```python
from build123d import *

# Parameters (mm, degrees)
SKETCH1_W           = 15
SKETCH1_H           = 4
BOSS_EXTRUDE1_DEPTH = 1
BOSS_EXTRUDE2_START = 6
BOSS_EXTRUDE2_DEPTH = 6
SKETCH3_W           = 10
SKETCH3_H           = 3
BOSS_EXTRUDE3_DEPTH = 3.5
BOSS_EXTRUDE4_START = 0.6
BOSS_EXTRUDE4_DEPTH = 0.6
SKETCH5_W           = 3
SKETCH5_H           = 10
BOSS_EXTRUDE5_DEPTH = 3.5


with BuildPart() as part:
    # Sketch1 → Boss-Extrude1 (new body)
    with BuildSketch(Plane(origin=(0, 0, 0), x_dir=(1, 0, 0), z_dir=(0, 1, 0))):
        with BuildLine():
            Line((-28, -26.5), (28, -26.5))
            ThreePointArc((28, -26.5), (35.071067812, -23.571067812), (38, -16.5))
            Line((38, -16.5), (38, 16.5))
            ThreePointArc((38, 16.5), (35.071067812, 23.571067812), (28, 26.5))
            Line((28, 26.5), (-28, 26.5))
            ThreePointArc((-28, 26.5), (-35.071067812, 23.571067812), (-38, 16.5))
            Line((-38, 16.5), (-38, -16.5))
            ThreePointArc((-38, -16.5), (-35.071067812, -23.571067812), (-28, -26.5))
        make_face()
        with Locations((16.5, 7)):
            Rectangle(SKETCH1_W, SKETCH1_H, mode=Mode.SUBTRACT)
    extrude(amount=BOSS_EXTRUDE1_DEPTH)

    # Sketch2 → Boss-Extrude2 (add)
    with BuildSketch(Plane.XZ.offset(BOSS_EXTRUDE2_START)):
        with BuildLine():
            Line((-28, -26.5), (28, -26.5))
            ThreePointArc((28, -26.5), (35.071067812, -23.571067812), (38, -16.5))
            Line((38, -16.5), (38, 16.5))
            ThreePointArc((38, 16.5), (35.071067812, 23.571067812), (28, 26.5))
            Line((28, 26.5), (-28, 26.5))
            ThreePointArc((-28, 26.5), (-35.071067812, 23.571067812), (-38, 16.5))
            Line((-38, 16.5), (-38, -16.5))
            ThreePointArc((-38, -16.5), (-35.071067812, -23.571067812), (-28, -26.5))
        make_face()
        with BuildLine():
            Line((28, 25.5), (-28, 25.5))
            ThreePointArc((-28, 25.5), (-34.363961031, 22.863961031), (-37, 16.5))
            Line((-37, 16.5), (-37, -16.5))
            ThreePointArc((-37, -16.5), (-34.363961031, -22.863961031), (-28, -25.5))
            Line((-28, -25.5), (28, -25.5))
            ThreePointArc((28, -25.5), (34.363961031, -22.863961031), (37, -16.5))
            Line((37, -16.5), (37, 16.5))
            ThreePointArc((37, 16.5), (34.363961031, 22.863961031), (28, 25.5))
        make_face(mode=Mode.SUBTRACT)
    extrude(amount=-BOSS_EXTRUDE2_DEPTH)

    # Sketch3 → Boss-Extrude3 (add)
    with BuildSketch(Plane.XZ):
        with Locations((0, -24)):
            Rectangle(SKETCH3_W, SKETCH3_H)
        with Locations((0, 24)):
            Rectangle(SKETCH3_W, SKETCH3_H)
    extrude(amount=BOSS_EXTRUDE3_DEPTH)

    # Sketch4 → Boss-Extrude4 (add)
    with BuildSketch(Plane.XZ.offset(6).offset(BOSS_EXTRUDE4_START)):
        with BuildLine():
            Line((-28, -26.5), (28, -26.5))
            ThreePointArc((28, -26.5), (35.071067812, -23.571067812), (38, -16.5))
            Line((38, -16.5), (38, 16.5))
            ThreePointArc((38, 16.5), (35.071067812, 23.571067812), (28, 26.5))
            Line((28, 26.5), (-28, 26.5))
            ThreePointArc((-28, 26.5), (-35.071067812, 23.571067812), (-38, 16.5))
            Line((-38, 16.5), (-38, -16.5))
            ThreePointArc((-38, -16.5), (-35.071067812, -23.571067812), (-28, -26.5))
        make_face()
        with BuildLine():
            Line((28, 25), (-28, 25))
            ThreePointArc((-28, 25), (-34.01040764, 22.51040764), (-36.5, 16.5))
            Line((-36.5, 16.5), (-36.5, -16.5))
            ThreePointArc((-36.5, -16.5), (-34.01040764, -22.51040764), (-28, -25))
            Line((-28, -25), (28, -25))
            ThreePointArc((28, -25), (34.01040764, -22.51040764), (36.5, -16.5))
            Line((36.5, -16.5), (36.5, 16.5))
            ThreePointArc((36.5, 16.5), (34.01040764, 22.51040764), (28, 25))
        make_face(mode=Mode.SUBTRACT)
    extrude(amount=-BOSS_EXTRUDE4_DEPTH)

    # Sketch5 → Boss-Extrude5 (add)
    with BuildSketch(Plane.XZ):
        with Locations((35.5, 0)):
            Rectangle(SKETCH5_W, SKETCH5_H)
        with Locations((-35.5, 0)):
            Rectangle(SKETCH5_W, SKETCH5_H)
    extrude(amount=BOSS_EXTRUDE5_DEPTH)


solid = part.part
```
Part model, mm, in its own coordinate system. A direction names the side the tool comes from. Round coordinates to 2 decimals unless told otherwise and drop trailing zeros. Write each loop counter-clockwise with the first axis right and the second up, starting at its lowest first coordinate (ties: lowest second). Pieces come first, ordered by that corner, then holes.
Item 1: Probe L1, parallel to Z at x = -23.5, y = -3.75; L2, parallel to X at y = -3.5, z = -8; L3, parallel to X at y = -3, z = -3.5. List the from-to ranges inside material, lowest first.
Results:
L1: z = -26.5 to -25.5, 25.5 to 26.5
L2: x = -38 to -37, 37 to 38
L3: x = -38 to -34, 34 to 38
Item 2: Cut at C-C, the plane x = 17.5. Give the cut face in (y, z).
Results:
outline: (-6.6, -26.5) - (1, -26.5) - (1, -9) - (0, -9) - (0, -25.5) - (-6, -25.5) - (-6, -25) - (-6.6, -25) - close; (-6.6, 25) - (-6, 25) - (-6, 25.5) - (0, 25.5) - (0, -5) - (1, -5) - (1, 26.5) - (-6.6, 26.5) - close
Item 3: Cut at D-D, the plane z = 7. Give the cut face in (x, y).
Results:
outline: (-38, -6.6) - (-36.5, -6.6) - (-36.5, -6) - (-37, -6) - (-37, 0) - (37, 0) - (37, -6) - (36.5, -6) - (36.5, -6.6) - (38, -6.6) - (38, 1) - (-38, 1) - close
Item 4: Two-plate mould, pull along X, no slides. Class faces 4 (the flat face through (-9, -6.6, 26)), 5 (the cylindrical face through (33.94, -6.3, -22.58)), 6 (the cylindrical face through (-34.99, -2.85, 23.65)): +X half, -X half, draft (parallel to the pull), parting line (faces both ways), or undercut.
Results:
face 4: draft
face 5: undercut
face 6: -X half
Item 5: Drop flat-ended pins along their axis: pin 1 Ø2.5 at (x, y) = (-35.5, -2) entering from +Z; pin 2 Ø1.5 at (y, z) = (-1, -23.5) entering from +X; pin 3 Ø0.9 at (y, z) = (-2, 24) entering from +X. Give the stop position or say it passes through.
Results:
pin 1: stops at z = 24.31
pin 2: stops at x = 35.81
pin 3: stops at x = 35.09
Item 6: Cut at A-A, the plane y = -4.25. Give the cut face in (x, z).
Results:
outline: (-38, -16.5) arc R10 ccw to (-28, -26.5) - (28, -26.5) arc R10 ccw to (38, -16.5) - (38, 16.5) arc R10 ccw to (28, 26.5) - (-28, 26.5) arc R10 ccw to (-38, 16.5) - close; hole (-37, -16.5) arc R9 ccw to (-28, -25.5) - (28, -25.5) arc R9 ccw to (37, -16.5) - (37, 16.5) arc R9 ccw to (28, 25.5) - (-28, 25.5) arc R9 ccw to (-37, 16.5) - close
Item 7: Which spindle directions (+Z, -Z, +X, -X, +Y, -Y) get a long thin tool onto all of the face, cutting with end or side? Do faces 1 (the flat face through (-36, -2, -5)), 2 (the flat face through (-34, -2, 0)), 3 (the flat face through (0, -3, -26.5)). Say none if no direction does.
Results:
face 1: none
face 2: -Y
face 3: -Z, +X, -X, +Y, -Y
Item 8: Cut at B-B, the plane z = -8. Give the cut face in (x, y), plus the area to 3 significant figures.
Results:
outline: (-38, -6.6) - (-36.5, -6.6) - (-36.5, -6) - (-37, -6) - (-37, 0) - (9, 0) - (9, 1) - (-38, 1) - close; (24, 0) - (37, 0) - (37, -6) - (36.5, -6) - (36.5, -6.6) - (38, -6.6) - (38, 1) - (24, 1) - close
area: 74.8 mm2
